Model file for the job. Use its own axes, mm. A direction names the side the tool comes from. Coordinates: 2 decimals unless noted, no trailing zeros. Loops run counter-clockwise (first coordinate to the right, second up) from the corner with the lowest first, then second, coordinate; pieces in that order, holes last. Notation, with made-up numbers: (-26.75, 44) -> (0.25, 44) arc R7 ccw to (0.25, 49) -> close; hole circle Ø4 at (59.5, -9). An arc over 180 degrees is marked (long way). Use one line per item in the form item = value.
```python
from build123d import *

# Parameters (mm, degrees)
SKETCH2_R          = 2.5
CUT_EXTRUDE1_DEPTH = 15.8
SKETCH3_R          = 1
CUT_EXTRUDE2_DEPTH = 7
SKETCH4_R          = 1.5
CUT_EXTRUDE3_DEPTH = 9


with BuildPart() as part:
    # Sketch1 → Revolve1 (revolve)
    with BuildSketch(Plane.XY):
        with BuildLine():
            Line((0, 7), (0, 3.9))
            ThreePointArc((0, 3.9), (0.029289322, 3.829289322), (0.1, 3.8))
            Line((0.1, 3.8), (0.3, 3.8))
            Line((0.3, 3.8), (0, 3.5))
            Line((0, 3.5), (0, 0))
            Line((0, 0), (14.8, 0))
            Line((14.8, 0), (14.8, 3.854253969))
            Line((14.8, 3.854253969), (14.3, 4.354253969))
            Line((14.3, 4.354253969), (13.887802139, 4.354253969))
            Line((13.887802139, 4.354253969), (13.887802139, 6.354253969))
            Line((13.887802139, 6.354253969), (14.710675154, 8))
            Line((14.710675154, 8), (13.710675154, 8))
            Line((13.710675154, 8), (13, 6.578649691))
            Line((13, 6.578649691), (6, 6.578649691))
            Line((6, 6.578649691), (6, 7))
            Line((6, 7), (5.5, 8))
            Line((5.5, 8), (0.5, 8))
            Line((0.5, 8), (0, 7))
        make_face()
    revolve(axis=Axis((0, 0, 0), (1, 0, 0)))

    # Sketch2 → Cut-Extrude1 (cut, through all)
    with BuildSketch(Plane(origin=(14.8, 0, 0), x_dir=(0, 0, -1), z_dir=(1, 0, 0))):
        Circle(SKETCH2_R)
    extrude(amount=-CUT_EXTRUDE1_DEPTH, mode=Mode.SUBTRACT)

    # Sketch3 → Cut-Extrude2 (cut)
    with BuildSketch(Plane(origin=(6, 0, 0), x_dir=(0, 0, -1), z_dir=(1, 0, 0))):
        with Locations((2.854369126, 5.927158565)):
            Circle(SKETCH3_R)
        with Locations((0, 6.578649691)):
            Circle(SKETCH3_R)
        with Locations((5.143395441, 4.101720992)):
            Circle(SKETCH3_R)
        with Locations((6.413709208, 1.463887273)):
            Circle(SKETCH3_R)
        with Locations((6.413709208, -1.463887273)):
            Circle(SKETCH3_R)
        with Locations((5.143395441, -4.101720992)):
            Circle(SKETCH3_R)
        with Locations((2.854369126, -5.927158565)):
            Circle(SKETCH3_R)
        with Locations((0, -6.578649691)):
            Circle(SKETCH3_R)
        with Locations((-2.854369126, -5.927158565)):
            Circle(SKETCH3_R)
        with Locations((-5.143395441, -4.101720992)):
            Circle(SKETCH3_R)
        with Locations((-6.413709208, -1.463887273)):
            Circle(SKETCH3_R)
        with Locations((-6.413709208, 1.463887273)):
            Circle(SKETCH3_R)
        with Locations((-5.143395441, 4.101720992)):
            Circle(SKETCH3_R)
        with Locations((-2.854369126, 5.927158565)):
            Circle(SKETCH3_R)
    extrude(amount=CUT_EXTRUDE2_DEPTH, mode=Mode.SUBTRACT)

    # Sketch4 → Cut-Extrude3 (cut, through all)
    with BuildSketch(Plane.XY):
        with Locations((3, 0)):
            Circle(SKETCH4_R)
    extrude(amount=CUT_EXTRUDE3_DEPTH, mode=Mode.SUBTRACT)


solid = part.part
```
Q1. Mould opens along Z. For faces 1 (the face through (2.96, -1.73, -7.81)), 2 (the face through (9.45, -2.85, 5.93)), 3 (the face through (14.09, -3.21, 2.94)) say: released by +Z, released by -Z, zero draft, split by the parting line, or undercut.
Result:
face_1 = split by the parting line
face_2 = released by +Z
face_3 = undercut
Q2. Wall check: line 1 along Z through (x, y) = (6.5, 0); line 2 along X through (y, z) = (-5.5, 2.5); line 3 along X through (y, z) = (-4.25, -1.5). Give the ranges that are in metal, low to high.
Result:
line_1 = -6.58 to -2.5, 2.5 to 6.58
line_2 = 0 to 6, 13 to 13.89
line_3 = 0 to 13.89
Q3. Band-saw the part on C-C, the plane x = 5.25. Write the cut outline in (y, z).
Result:
outline = circle Ø16 at (0, 0); hole circle Ø5 at (0, 0)
Q4. Pin check, flat tips, straight feed: pin 1 Ø6 at (x, y) = (12.5, 5.5) entering from -Z; pin 2 Ø5 at (x, y) = (7.5, 3) entering from +Z. Stop position of each tip, or through.
Result:
pin_1 = -7.51
pin_2 = 7.86
Q5. Band-saw the part on D-D, the plane x = 3. Write the cut outline in (y, z).
Result:
outline = (-1.5, 2) -> (-1.5, 7.86) arc R8 ccw (long way) to (1.5, 7.86) -> (1.5, 2) arc R2.5 cw (long way) to start
Q6. Band-saw the part on B-B, the plane y = 0. State how many separate pieces and enclosed holes the cut face has, and give its area (3 significant figures).
Result:
separate_pieces = 3
enclosed_holes = 0
area = 119 mm2
Q7. Which spindle directions (+Z, -Z, +X, -X, +Y, -Y) get a long thin tool onto all of the face, cutting with end or side? Do faces 4 (the face through (9.451, 6.415, 1.457)), 5 (the face through (13, -6, 0)), 6 (the face through (9.451, -6.412, 1.47)). Say none if no direction does.
Result:
face_4 = +Z, +Y
face_5 = -Y
face_6 = +Z, -Y
